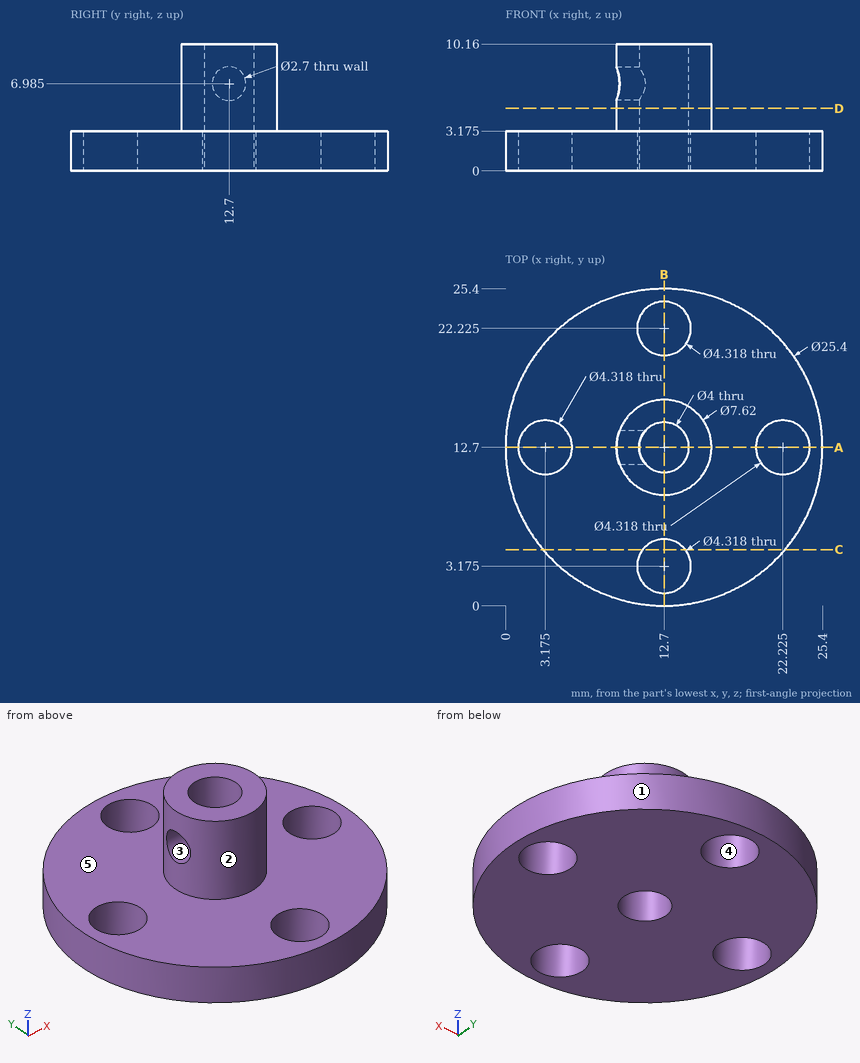
Geometry: see drawing. Coordinates: mm, zero at the bounding-box minimum. A direction names the side the tool comes from. Round coordinates to 2 decimals unless told otherwise and drop trailing zeros. Order: outer loops, then holes, each group sorted by start corner. A loop starts at its lowest first (then second) coordinate and runs counter-clockwise, first axis right, second up. Notation, with made-up numbers: (43.5, 67.5) -> (53.5, 67.5) arc R20 ccw to (53.5, 82.5) -> close; hole circle Ø7 at (77.25, 69). An arc over 180 degrees is marked (long way). Use CSV: the item, a comma, the result in double quotes.
(1) Section C-C on y = 4.5. Return the cut outline in (x, z) (3 decimals), and give its area (3 significant figures).
Report:
outline,"(3.002, 0) -> (10.995, 0) -> (10.995, 3.175) -> (3.002, 3.175) -> close; (14.405, 0) -> (22.398, 0) -> (22.398, 3.175) -> (14.405, 3.175) -> close"
area,"50.8 mm^2"
(2) Section A-A on y = 12.7. Return the cut outline in (x, z) (3 decimals).
Report:
outline,"(0, 0) -> (1.016, 0) -> (1.016, 3.175) -> (0, 3.175) -> close; (5.334, 0) -> (10.7, 0) -> (10.7, 5.635) -> (8.89, 5.635) -> (8.89, 3.175) -> (5.334, 3.175) -> close; (8.89, 8.335) -> (10.7, 8.335) -> (10.7, 10.16) -> (8.89, 10.16) -> close; (14.7, 0) -> (20.066, 0) -> (20.066, 3.175) -> (16.51, 3.175) -> (16.51, 10.16) -> (14.7, 10.16) -> close; (24.384, 0) -> (25.4, 0) -> (25.4, 3.175) -> (24.384, 3.175) -> close"
(3) Section D-D on z = 5. Return the cut outline in (x, y).
Report:
outline,"circle Ø7.62 at (12.7, 12.7); hole circle Ø4 at (12.7, 12.7)"
(4) First-contact query: pin 1 Ø4 at (x, z) = (14, 3) entering from -Y; pin 2 Ø3.5 at (y, z) = (12.7, 6.985) entering from -X; pin 3 Ø6 at (y, z) = (20, 6.5) entering from -X; pin 4 Ø1 at (y, z) = (3, 2.5) entering from +X (3 decimals). Flat tips, straight axial feed; report the tip coordinate or a pass-through.
Report:
pin 1,"y = 0"
pin 2,"x = 8.89"
pin 3,"through"
pin 4,"x = 21.455"
(5) Pull-direction query (Z, two-part tool) for the marked faces 3, 4 and 5; classes: +Z half, -Z half, draft (parallel to the pull), parting line (faces both ways), or undercut.
Report:
face 3,"undercut"
face 4,"draft"
face 5,"+Z half"
(6) Access query for the marked faces 1 and 2. Directions: +Z, -Z, +X, -X, +Y, -Y. A direction counts if a zero-diameter tool reaches every point of the face in a straight line with its end or side. Return the directions, or none.
Report:
face 1,"+Z, -Z"
face 2,"+Z"
(7) Section B-B on x = 12.7. Return the cut outline in (y, z) (3 decimals), and give its area (3 significant figures).
Report:
outline,"(0, 0) -> (1.016, 0) -> (1.016, 3.175) -> (0, 3.175) -> close; (5.334, 0) -> (10.7, 0) -> (10.7, 10.16) -> (8.89, 10.16) -> (8.89, 3.175) -> (5.334, 3.175) -> close; (14.7, 0) -> (20.066, 0) -> (20.066, 3.175) -> (16.51, 3.175) -> (16.51, 10.16) -> (14.7, 10.16) -> close; (24.384, 0) -> (25.4, 0) -> (25.4, 3.175) -> (24.384, 3.175) -> close"
area,"65.8 mm^2"
(8) Ray query, L1, parallel to X at y = 12.7, z = 3.25; L2, parallel to X at y = 14, z = 2.5; L3, parallel to Z at x = 8, y = 6.5 (3 decimals). Return the intervals inside material, ascending.
Report:
L1,"8.89 to 10.7, 14.7 to 16.51"
L2,"0.07 to 1.45, 4.9 to 11.18, 14.22 to 20.5, 23.95 to 25.33"
L3,"0 to 3.175"
